Design review of the part built by this model. Coordinates are the model's own, in mm. Face numbers are marked on the shaded views. A direction names the side the tool comes from. Coordinates: 2 decimals unless noted, no trailing zeros. Write each loop counter-clockwise with the first axis right and the second up, starting at its lowest first coordinate (ties: lowest second). Pieces come first, ordered by that corner, then holes.
Q1. Add section C-C, the plane y = 8. Give the boundary of the cut face in (x, z) (3 decimals), plus the area to 3 significant figures.
Q2. The part is to be moulded in two halves that separate along X. For the marked faces 5, 6 and 7, say which applies: +X half, -X half, draft (parallel to the pull), parting line (faces both ways), or undercut.
Q3. To check wall thickness, follow probe 1 along Y at (x, z) = (18.5, 6.5); probe 2 along Y at (x, z) = (10, 15); probe 3 along Z at (x, y) = (0, 25) (3 decimals). State the ranges of each line that lie inside material, in increasing order.
Q4. Add section A-A, the plane y = 20.5. Give the boundary of the cut face in (x, z) (3 decimals), plus the area to 3 significant figures.
Q5. Add section B-B, the plane x = 0. Give the number of separate pieces and of enclosed holes in the cut face, plus the area to 3 significant figures.
Q6. Clearance check with flat-ended pins moving along their axes: pin 1 Ø3.5 at (y, z) = (17, 14.5) entering from +X; pin 2 Ø6 at (x, y) = (-3.5, 25) entering from +Z; pin 3 Ø12.5 at (x, z) = (3, 8) entering from +Y. State where each tip first meets the part, or that it passes through.
Q7. Machinability: for the marked faces 1, 2, 3 and 4, which of the approach directions +Z, -Z, +X, -X, +Y, -Y give a long, thin tool a straight path to every point of the face, cutting with its end or side? Answer none if there is none.
from build123d import *

# Parameters (mm, degrees)
CHAMFER1_SIZE           = 3
CHAMFER2_SIZE           = 0.5
SKETCH2_R               = 4
CUT_EXTRUDE1_DEPTH      = 43
SKETCH3_W               = 1.5
SKETCH3_H               = 21.5
CUT_EXTRUDE2_DEPTH      = 21.9
CUT_EXTRUDE2_DEPTH_BACK = 21.9
CUT_EXTRUDE3_DEPTH      = 6.5
CUT_EXTRUDE3_DEPTH_BACK = 37.3


with BuildPart() as part:
    # Sketch1 → Revolve1 (revolve)
    with BuildSketch(Plane.XY, mode=Mode.PRIVATE) as revolve1_sk:
        Polygon((0, 0), (12.475, 0), (12.475, 35), (20.9, 35), (20.9, 33), (18.1, 33), (18.1, 29.5), (20.9, 29.5), (20.9, 27.5), (16.9, 27.5), (16.9, 0.5), (20.9, 0.5), (20.9, -1.5), (18.1, -1.5), (18.1, -5), (20.9, -5), (20.9, -7), (0, -7), align=None)
    revolve(revolve1_sk.sketch.rotate(Axis((0, 0, 0), (0, -1, 0)), 180), axis=Axis((0, 0, 0), (0, -1, 0)))  # turned: the seam where the file's is

    # Chamfer1
    chamfer1_edges = [part.edges().sort_by_distance(p)[0] for p in [
        (12.475, 35, 0),
    ]]
    chamfer(chamfer1_edges, length=CHAMFER1_SIZE)

    # Chamfer2
    chamfer2_edges = [part.edges().sort_by_distance(p)[0] for p in [
        (20.9, 35, 0),
        (20.9, -7, 0),
    ]]
    chamfer(chamfer2_edges, length=CHAMFER2_SIZE)

    # Sketch2 → Cut-Extrude1 (cut, through all)
    with BuildSketch(Plane.XZ.offset(7)):
        Circle(SKETCH2_R)
    extrude(amount=-CUT_EXTRUDE1_DEPTH, mode=Mode.SUBTRACT)

    # Sketch3 → Cut-Extrude2 (cut, two sides)
    with BuildSketch(Plane(origin=(0, 0, 0), x_dir=(0, 0, -1), z_dir=(1, 0, 0))) as cut_extrude2_sk:
        with Locations((16.15, 16.75)):
            Rectangle(SKETCH3_W, SKETCH3_H)
        with Locations((-16.15, 16.75)):
            Rectangle(SKETCH3_W, SKETCH3_H)
    extrude(amount=CUT_EXTRUDE2_DEPTH, mode=Mode.SUBTRACT)
    extrude(cut_extrude2_sk.sketch, amount=-CUT_EXTRUDE2_DEPTH_BACK, mode=Mode.SUBTRACT)

    # Sketch4 → Cut-Extrude3 (cut, two sides)
    with BuildSketch(Plane.XY.offset(15.4)) as cut_extrude3_sk:
        with BuildLine():
            Line((4, 18.3), (4, 15))
            ThreePointArc((4, 15), (0, 11), (-4, 15))
            Line((-4, 15), (-4, 18.3))
            ThreePointArc((-4, 18.3), (0, 22.3), (4, 18.3))
        make_face()
    extrude(amount=CUT_EXTRUDE3_DEPTH, mode=Mode.SUBTRACT)
    extrude(cut_extrude3_sk.sketch, amount=-CUT_EXTRUDE3_DEPTH_BACK, mode=Mode.SUBTRACT)


solid = part.part
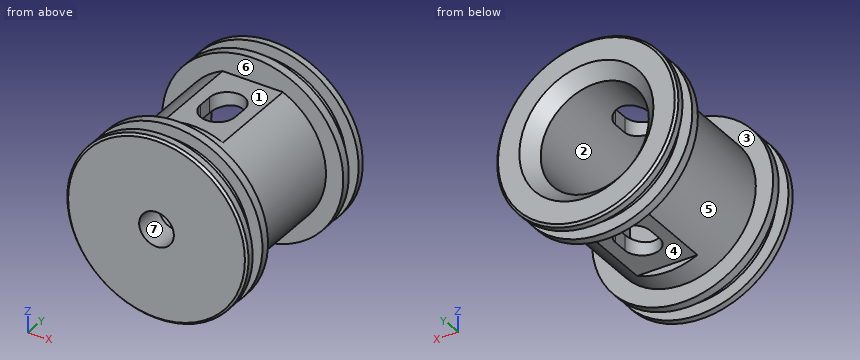
Here are the results:
1. outline: (-6.961, -15.4) - (6.961, -15.4) arc R16.9 ccw to (6.961, 15.4) - (-6.961, 15.4) arc R16.9 ccw to start; hole circle Ø24.95 at (0, 0)
1. area: 380 mm2
2. face 5: parting line
2. face 6: draft
2. face 7: undercut
3. probe 1: y = -7 to -5, -1.5 to 0.5, 27.5 to 29.5, 33 to 35
3. probe 2: y = -7 to 0.5, 27.5 to 35
3. probe 3: z = -15.4 to -12.475, 12.475 to 15.4
4. outline: (-6.961, -15.4) - (-3.341, -15.4) - (-3.341, -12.019) arc R12.475 cw to (-3.341, 12.019) - (-3.341, 15.4) - (-6.961, 15.4) arc R16.9 ccw to start; (3.341, -15.4) - (6.961, -15.4) arc R16.9 ccw to (6.961, 15.4) - (3.341, 15.4) - (3.341, 12.019) arc R12.475 cw to (3.341, -12.019) - close
4. area: 339 mm2
5. separate pieces: 4
5. enclosed holes: 0
5. area: 431 mm2
6. pin 1: stops at x = 11.09
6. pin 2: stops at z = 20.82
6. pin 3: stops at y = 34.32
7. face 1: +Z, +X, -X
7. face 2: +Y
7. face 3: none
7. face 4: -Z, +X, -X
